For this review, take the finished solid that the model builds, in its own axes (mm). A direction names the side the tool comes from. Round coordinates to 2 decimals unless told otherwise and drop trailing zeros. Loops run counter-clockwise (first coordinate to the right, second up) from the corner with the lowest first, then second, coordinate; pieces in that order, holes last.
1) Tool access review of faces 5 (the flat face through (500, -10, -62)), 6 (the flat face through (500, -10, 64)), 7 (the flat face through (-532, 4, -125)): name each direction out of +Z, -Z, +X, -X, +Y, -Y from which nothing blocks a thin tool from reaching the whole face with its end or side.
2) Take a section at C-C (x = -388.5). State the section outline as (y, z) points, then the cut area to 3 significant figures.
3) Take a section at A-A (z = 108). State the section outline as (x, y) points, then the cut area to 3 significant figures.
4) Mouldability with a two-part tool opening along X and no side actions: class faces 1 (the flat face through (-8, 750, 2)), 2 (the flat face through (-550, -10, 2)), 3 (the flat face through (550, -10, 2)), 4 (the flat face through (-7, 700, 64)) as pulls with the +X half, pulls with the -X half, needs draft (parallel to the pull), parting line crosses it, or undercut.
5) Take a section at B-B (y = 532.5). State the section outline as (x, z) points.
6) Wall thickness on L1, parallel to X at y = 93.5, z = -44.5; L2, parallel to Y at x = -168, z = -53.5; L3, parallel to Z at x = 411, y = 76: over which ranges is each line inside the solid? List them lowest first.
7) Insertion check: pin 1 (5 mm diameter, centred on x = 84, y = -308.5, fed in from -Z); pin 2 (8 mm diameter, centred on x = 290, y = -236, fed in from +Z). Each pin has a flat end and moves straight along its axis. Give the tip position at first contact, or say it passes through.
```python
from build123d import *

# Parameters (mm, degrees)
F0_W     = 1100
F0_H     = 1500
F0_W_2   = 1000
F0_H_2   = 1400
F1_DEPTH = 125
F2_W     = 1000
F2_H     = 1400
F3_DEPTH = 1.5


with BuildPart() as f1:
    # F0 (on Top) → F1 (new body, symmetric)
    with BuildSketch(Plane.XY):
        Rectangle(F0_W, F0_H)
        Rectangle(F0_W_2, F0_H_2, mode=Mode.SUBTRACT)
    extrude(amount=F1_DEPTH, both=True)

    # F2 (on Top) → F3 (join, symmetric)
    with BuildSketch(Plane.XY):
        Rectangle(F2_W, F2_H)
    extrude(amount=F3_DEPTH, both=True)


solid = f1.part
```
Response:
1. face 5: -Z
1. face 6: +Z
1. face 7: -Z, +X, -X, +Y, -Y
2. outline: (-750, -125) - (-700, -125) - (-700, -1.5) - (700, -1.5) - (700, -125) - (750, -125) - (750, 125) - (700, 125) - (700, 1.5) - (-700, 1.5) - (-700, 125) - (-750, 125) - close
2. area: 29,200 mm2
3. outline: (-550, -750) - (550, -750) - (550, 750) - (-550, 750) - close; hole (-500, -700) - (500, -700) - (500, 700) - (-500, 700) - close
3. area: 250,000 mm2
4. face 1: needs draft
4. face 2: pulls with the -X half
4. face 3: pulls with the +X half
4. face 4: undercut
5. outline: (-550, -125) - (-500, -125) - (-500, -1.5) - (500, -1.5) - (500, -125) - (550, -125) - (550, 125) - (500, 125) - (500, 1.5) - (-500, 1.5) - (-500, 125) - (-550, 125) - close
6. L1: x = -550 to -500, 500 to 550
6. L2: y = -750 to -700, 700 to 750
6. L3: z = -1.5 to 1.5
7. pin 1: stops at z = -1.5
7. pin 2: stops at z = 1.5
